For this review, take the finished solid that the model builds, in its own axes (mm). Face numbers are marked on the shaded views. A direction names the side the tool comes from. Round coordinates to 2 decimals unless told otherwise and drop trailing zeros. Write each loop counter-clockwise with the first axis right and the second up, starting at its lowest first coordinate (ties: lowest second). Pieces come first, ordered by that corner, then holes. Notation, with made-up numbers: (20.5, 65) -> (79.5, 65) arc R10 cw to (79.5, 82) -> close; hole circle Ø10 at (-9, 73). An arc over 180 degrees is marked (long way). Answer in a Markdown table with one row per item. Add a question column.
```python
from build123d import *

# Parameters (mm, degrees)
SKETCH1_R                            = 30
SKETCH1_R_2                          = 25.4
BOSS_EXTRUDE1_DEPTH                  = 203.2
SKETCH2_W                            = 12.7
SKETCH2_H                            = 63.5
BOSS_EXTRUDE2_DEPTH                  = 50.8
BOSS_EXTRUDE2_DIRECTION_2_REACH      = 215.987
BOSS_EXTRUDE2_DIRECTION_2_END_RADIUS = 30
CUT_EXTRUDE3_REACH                   = 223.676
SKETCH3_R                            = 6.35
CUT_EXTRUDE3_DIRECTION_2_DEPTH       = 222.675895171


with BuildPart() as part:
    # Sketch1 → Boss-Extrude1 (new body)
    with BuildSketch(Plane(origin=(0, 0, 0), x_dir=(1, 0, 0), z_dir=(0, 1, 0))):
        with Locations(Location((0, 0, 0), (0, 0, 270))):
            Circle(SKETCH1_R)
        with Locations(Location((0, 0, 0), (0, 0, 270))):
            Circle(SKETCH1_R_2, mode=Mode.SUBTRACT)
    extrude(amount=BOSS_EXTRUDE1_DEPTH)

    # Sketch2 → Boss-Extrude2 (add)
    with BuildSketch(Plane(origin=(0, 0, -30), x_dir=(-1, 0, 0), z_dir=(0, 0, -1))):
        with Locations((0, 101.6)):
            Rectangle(SKETCH2_W, SKETCH2_H)
    extrude(amount=BOSS_EXTRUDE2_DEPTH)

    # Boss-Extrude2 direction 2: up to this cylinder (the profile starts outside it)
    boss_extrude2_direction_2_end = Plane(origin=(0, 101.6, 0), z_dir=(0, -1, 0)) * Cylinder(BOSS_EXTRUDE2_DIRECTION_2_END_RADIUS, 492.974, mode=Mode.PRIVATE)
    # Sketch2 → Boss-Extrude2 direction 2 (add, up to the surface)
    with BuildSketch(Plane(origin=(0, 0, -30), x_dir=(-1, 0, 0), z_dir=(0, 0, -1)), mode=Mode.PRIVATE) as boss_extrude2_direction_2_sk1:
        with Locations((0, 101.6)):
            Rectangle(SKETCH2_W, SKETCH2_H)
    boss_extrude2_direction_2_tool1 = extrude(boss_extrude2_direction_2_sk1.sketch, amount=-BOSS_EXTRUDE2_DIRECTION_2_REACH, mode=Mode.PRIVATE) - boss_extrude2_direction_2_end
    add(boss_extrude2_direction_2_tool1.solids().sort_by_distance((0, 101.6, -30))[0])
    add(boss_extrude2_direction_2_tool1.solids().sort_by_distance((0, 101.6, -30))[1])

    # Sketch3 → Cut-Extrude3 (cut, up to next)
    with BuildSketch(Plane(origin=(6.35, 0, 0), x_dir=(0, 0, -1), z_dir=(1, 0, 0)), mode=Mode.PRIVATE) as cut_extrude3_sk1:
        with BuildLine():
            Line((72.678913322, 93.247804014), (30, 69.85))
            Line((30, 69.85), (80.8, 69.85))
            Line((80.8, 69.85), (80.8, 133.35))
            Line((80.8, 133.35), (30, 133.35))
            Line((30, 133.35), (72.678913322, 109.952195986))
            ThreePointArc((72.678913322, 109.952195986), (76.295723714, 106.453425368), (77.625, 101.6))
            ThreePointArc((77.625, 101.6), (76.295723714, 96.746574632), (72.678913322, 93.247804014))
        make_face()
    cut_extrude3_tool1 = extrude(cut_extrude3_sk1.sketch, amount=-CUT_EXTRUDE3_REACH, mode=Mode.PRIVATE) & part.part
    # Sketch3 → Cut-Extrude3 (cut, up to next)
    with BuildSketch(Plane(origin=(6.35, 0, 0), x_dir=(0, 0, -1), z_dir=(1, 0, 0)), mode=Mode.PRIVATE) as cut_extrude3_sk2:
        with Locations((68.1, 101.6)):
            Circle(SKETCH3_R)
    cut_extrude3_tool2 = extrude(cut_extrude3_sk2.sketch, amount=-CUT_EXTRUDE3_REACH, mode=Mode.PRIVATE) & part.part
    add(cut_extrude3_tool1.solids().sort_by_distance((6.35, 80.835833, -51.730381))[0], mode=Mode.SUBTRACT)
    add(cut_extrude3_tool2.solids().sort_by_distance((6.35, 101.6, -68.1))[0], mode=Mode.SUBTRACT)

    # Sketch3 → Cut-Extrude3 direction 2 (cut)
    with BuildSketch(Plane(origin=(6.35, 0, 0), x_dir=(0, 0, -1), z_dir=(1, 0, 0))):
        with BuildLine():
            Line((72.678913322, 93.247804014), (30, 69.85))
            Line((30, 69.85), (80.8, 69.85))
            Line((80.8, 69.85), (80.8, 133.35))
            Line((80.8, 133.35), (30, 133.35))
            Line((30, 133.35), (72.678913322, 109.952195986))
            ThreePointArc((72.678913322, 109.952195986), (76.295723714, 106.453425368), (77.625, 101.6))
            ThreePointArc((77.625, 101.6), (76.295723714, 96.746574632), (72.678913322, 93.247804014))
        make_face()
        with Locations((68.1, 101.6)):
            Circle(SKETCH3_R)
    extrude(amount=CUT_EXTRUDE3_DIRECTION_2_DEPTH, mode=Mode.SUBTRACT)


solid = part.part
```
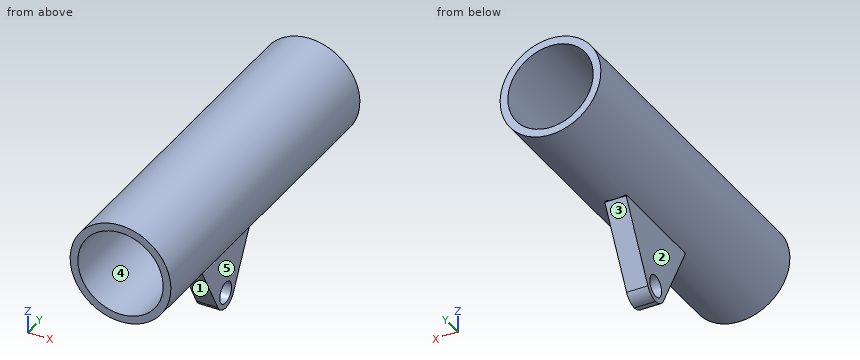
1. We need section C-C (z = -12.5). Write out the cut boundary in (x, y).
2. We need section B-B (y = 37). Write out the cut boundary in (x, z).
3. We need section A-A (z = 0). Write out the cut boundary in (x, y).
4. The part is to be moulded in two halves that separate along X. For the marked faces 3, 4 and 5, say which applies: pulls with the +X half, pulls with the -X half, needs draft (parallel to the pull), parting line crosses it, or undercut.
5. Clearance check with flat-ended pins moving along their axes: pin 1 Ø24 at (y, z) = (108, -45.5) entering from -X; pin 2 Ø8 at (y, z) = (99, -16.5) entering from -X; pin 3 Ø12 at (x, y) = (-22, 156) entering from -Z; pin 4 Ø8 at (x, z) = (-14.5, 18.5) entering from +Y. State where each tip first meets the part, or that it passes through.
6. For L1, parallel to X at y = 117, z = 0; L2, parallel to X at y = 67, z = -17; L3, parallel to Y at x = -5, z = -71, list the stretches that pass through material, from the lowest coordinate up. Write a range as [from, to].
7. Tool access review of the marked faces 1 and 2: name each direction out of +Z, -Z, +X, -X, +Y, -Y from which nothing blocks a thin tool from reaching the whole face with its end or side.
8. We need section D-D (z = -56.5). Write out the cut boundary in (x, y).
Response:
| question | item | result |
|---|---|---|
| 1 | outline | (-27.27, 0) -> (-22.11, 0) -> (-22.11, 203.2) -> (-27.27, 203.2) -> close; (22.11, 0) -> (27.27, 0) -> (27.27, 203.2) -> (22.11, 203.2) -> close |
| 2 | outline | circle Ø60 at (0, 0); hole circle Ø50.8 at (0, 0) |
| 3 | outline | (-30, 0) -> (-25.4, 0) -> (-25.4, 203.2) -> (-30, 203.2) -> close; (25.4, 0) -> (30, 0) -> (30, 203.2) -> (25.4, 203.2) -> close |
| 4 | face 3 | needs draft |
| 4 | face 4 | undercut |
| 4 | face 5 | pulls with the +X half |
| 5 | pin 1 | x = -6.35 |
| 5 | pin 2 | x = -27.27 |
| 5 | pin 3 | z = -25.38 |
| 5 | pin 4 | y = 203.2 |
| 6 | L1 | [-30, -25.4], [25.4, 30] |
| 6 | L2 | [-24.72, -18.87], [18.87, 24.72] |
| 6 | L3 | [92.33, 95.95], [107.25, 110.87] |
| 7 | face 1 | -Z, +X, -X, -Y |
| 7 | face 2 | -Z, -X, +Y, -Y |
| 8 | outline | (-6.35, 84.38) -> (6.35, 84.38) -> (6.35, 118.82) -> (-6.35, 118.82) -> close |
